```python
from build123d import *

# Parameters (mm, degrees)
SKETCH1_R           = 7
BOSS_EXTRUDE1_DEPTH = 4


with BuildPart() as part:
    # Sketch1 → Boss-Extrude1 (new body)
    with BuildSketch(Plane(origin=(0, 0, 0), x_dir=(0, 0, -1), z_dir=(1, 0, 0))):
        with BuildLine():
            Line((-12.7, 0), (-12.7, 48.71))
            ThreePointArc((-12.7, 48.71), (-9.771067812, 55.781067812), (-2.7, 58.71))
            Line((-2.7, 58.71), (2.7, 58.71))
            ThreePointArc((2.7, 58.71), (9.771067812, 55.781067812), (12.7, 48.71))
            Line((12.7, 48.71), (12.7, 0))
            ThreePointArc((12.7, 0), (0, 12.7), (-12.7, 0))
        make_face()
        with Locations((0, 46.01)):
            Circle(SKETCH1_R, mode=Mode.SUBTRACT)
    extrude(amount=BOSS_EXTRUDE1_DEPTH)


solid = part.part
```
CAD build for the part. Positions are in the model's coordinates, mm. Coordinates: 2 decimals unless noted, no trailing zeros. Order: outer loops, then holes, each group sorted by start corner. A loop starts at its lowest first (then second) coordinate and runs counter-clockwise, first axis right, second up. Notation, with made-up numbers: (-14, 0.25) - (4, 0.25) arc R17 ccw to (4, 18.25) - close; hole circle Ø10 at (15, 4). An arc over 180 degrees is marked (long way). Use a Markdown table: item, result. Add a question column.
(1) Flat gauge pins, fed straight in: pin 1 (1 mm diameter, centred on x = 0.5, z = 7.5, fed in from +Y); pin 2 (8.5 mm diameter, centred on y = 46.01, z = 0, fed in from +X). Where does each tip first touch, or does it go through?
(2) Saw through at B-B (y = 46.01). Give the cut face in (x, z), then the cut area to 3 significant figures.
(3) Drill centre lines: line 1 along Y through (x, z) = (2.8, 0); line 2 along Z through (x, y) = (0.9, 7); line 3 along Y through (x, z) = (1.8, -2.5). Where is each one in solid material? Low to high. Write a range as [from, to].
(4) Saw through at A-A (z = 0). Give the cut face in (x, y), then the cut area to 3 significant figures.
(5) Pull direction Z, two halves, no side cores. Call faces 1 (the face through (2, 24, 12.7)), 2 (the face through (1.972, 51.912, -3.763)), 3 (the face through (1.972, 12.697, -0.279)), 4 (the face through (0, 30, 0)): +Z half, -Z half, draft (parallel to the pull), parting line (faces both ways), or undercut.
(6) Saw through at D-D (z = 9.5). Give the cut face in (x, y), then the cut area to 3 significant figures.
(7) Saw through at C-C (x = 1.05). Give the cut face in (y, z).
Solved:
| question | item | result |
|---|---|---|
| 1 | pin 1 | stops at y = 57.74 |
| 1 | pin 2 | passes through |
| 2 | outline | (0, -12.7) - (4, -12.7) - (4, -7) - (0, -7) - close; (0, 7) - (4, 7) - (4, 12.7) - (0, 12.7) - close |
| 2 | area | 45.6 mm² |
| 3 | line 1 | y = [12.7, 39.01], [53.01, 58.71] |
| 3 | line 2 | z = [-12.7, -10.6], [10.6, 12.7] |
| 3 | line 3 | y = [12.45, 39.47], [52.55, 58.71] |
| 4 | outline | (0, 12.7) - (4, 12.7) - (4, 39.01) - (0, 39.01) - close; (0, 53.01) - (4, 53.01) - (4, 58.71) - (0, 58.71) - close |
| 4 | area | 128 mm² |
| 5 | face 1 | +Z half |
| 5 | face 2 | undercut |
| 5 | face 3 | undercut |
| 5 | face 4 | draft |
| 6 | outline | (0, 8.43) - (4, 8.43) - (4, 56.04) - (0, 56.04) - close |
| 6 | area | 190 mm² |
| 7 | outline | (0, -12.7) - (48.71, -12.7) arc R10 ccw to (58.71, -2.7) - (58.71, 2.7) arc R10 ccw to (48.71, 12.7) - (0, 12.7) arc R12.7 cw to start; hole circle Ø14 at (46.01, 0) |
